The listing builds one solid part. Answer for the finished solid, in the listing's coordinates (mm). Round coordinates to 2 decimals unless told otherwise and drop trailing zeros. Write each loop counter-clockwise with the first axis right and the second up, starting at its lowest first coordinate (ties: lowest second). Pieces come first, ordered by that corner, then holes. Notation, with made-up numbers: M 87,-16 L 106,-16 A23 cw 106,9 Z; hole C 76,-9 d9. An arc over 180 degrees is marked long. Write each question's results on one line, items separated by ' | '.
from build123d import *

# Parameters (mm, degrees)
BOSS_EXTRUDE1_DEPTH = 79
FILLET1_R           = 2


with BuildPart() as part:
    # Sketch1 → Boss-Extrude1 (new body)
    with BuildSketch(Plane.XY):
        with BuildLine():
            Line((0, 0), (0, 9))
            ThreePointArc((0, 9), (-9, 0), (0, -9))
            Line((0, -9), (0, 0))
        make_face()
        with BuildLine():
            ThreePointArc((9, 0), (6.363961031, 6.363961031), (0, 9))
            Line((0, 9), (0, 0))
            Line((0, 0), (9, 0))
        make_face()
        with BuildLine():
            Line((19, 9), (0, 9))
            ThreePointArc((0, 9), (6.363961031, 6.363961031), (9, 0))
            Line((9, 0), (10, 0))
            ThreePointArc((10, 0), (12.636038969, 6.363961031), (19, 9))
        make_face()
        with BuildLine():
            Line((19, 0), (19, 9))
            ThreePointArc((19, 9), (12.636038969, 6.363961031), (10, 0))
            Line((10, 0), (19, 0))
        make_face()
        with BuildLine():
            ThreePointArc((28, 0), (25.363961031, 6.363961031), (19, 9))
            Line((19, 9), (19, 0))
            Line((19, 0), (19, -9))
            ThreePointArc((19, -9), (25.363961031, -6.363961031), (28, 0))
        make_face()
        with BuildLine():
            Line((19, -9), (19, 0))
            Line((19, 0), (10, 0))
            ThreePointArc((10, 0), (12.636038969, -6.363961031), (19, -9))
        make_face()
        with BuildLine():
            Line((10, 0), (9, 0))
            ThreePointArc((9, 0), (6.363961031, -6.363961031), (0, -9))
            Line((0, -9), (19, -9))
            ThreePointArc((19, -9), (12.636038969, -6.363961031), (10, 0))
        make_face()
        with BuildLine():
            Line((9, 0), (0, 0))
            Line((0, 0), (0, -9))
            ThreePointArc((0, -9), (6.363961031, -6.363961031), (9, 0))
        make_face()
    extrude(amount=BOSS_EXTRUDE1_DEPTH)

    # Fillet1
    fillet1_edges = [part.edges().sort_by_distance(p)[0] for p in [
        (9.5, 9, 79),
        (-9, 0, 79),
        (9.5, -9, 79),
        (-9, 0, 0),
        (9.5, 9, 0),
        (28, 0, 0),
        (9.5, -9, 0),
        (28, 0, 79),
    ]]
    fillet(fillet1_edges, radius=FILLET1_R)


solid = part.part
1) Section A-A (z = 45) is taken. Determine the outline of the cut face in (x, y), then the cut area to 3 significant figures.
Return value:
outline: M 0,-9 L 19,-9 A9 ccw 19,9 L 0,9 A9 ccw Z | area: 596 mm²
2) Find the intervals of material crossed by line 1 (X direction, y = -5.75, z = 65.5); line 2 (X direction, y = 6.25, z = 12); line 3 (Y direction, x = 25, z = 72.5), in increasing order.
Return value:
line 1: -6.92 to 25.92 | line 2: -6.48 to 25.48 | line 3: -6.71 to 6.71
3) Each of these flat-tipped pins is pushed along its axis until it touches: pin 1 (10 mm diameter, centred on y = -0.5, z = 33, fed in from -X); pin 2 (1 mm diameter, centred on x = 22, z = 19.5, fed in from -Y); pin 3 (1 mm diameter, centred on y = 5, z = 12.5, fed in from +X); pin 4 (4 mm diameter, centred on x = 22.5, z = 52.5, fed in from +Y). Where does it stop, or does it pass through?
Return value:
pin 1: x = -9 | pin 2: y = -8.65 | pin 3: x = 26.79 | pin 4: y = 8.87
